Autodesk Inventor part; units mm, degrees
ref_plane "YZ Plane" through (0, 0, 0) normal (1, 0, 0) x (0, 1, 0)
ref_plane "XZ Plane" through (0, 0, 0) normal (0, 1, 0) x (-1, 0, 0)
ref_plane "XY Plane" through (0, 0, 0) normal (0, 0, 1) x (1, 0, 0)
sketch "card" plane through (0, 0, 0) normal (0, 0, 1) x (1, 0, 0)
  line L0 (-59.3579, 68.5808) -> (-59.3579, 10.0008)
  line L1 (-59.3579, 10.0008) -> (14.2921, 10.0008)
  line L2 (14.2921, 10.0008) -> (14.2921, 68.5808)
  line L3 (14.2921, 68.5808) -> (-59.3579, 68.5808)
  circle A0 centre (11.6671, 65.9558) radius 1.575
  circle A1 centre (11.6671, 12.6258) radius 1.575
  circle A2 centre (-56.7329, 65.9558) radius 1.575
  circle A3 centre (-56.7329, 12.6258) radius 1.575
  point P0 (0, 0)
  dimension "d1" = 58.58
  dimension "d2" = 73.65
  dimension "d4" = 2.625
  dimension "d5" = 3.15
extrude "main_board" add sketch "card" along normal blind 1.6
sketch "back_components" plane through (0, 0, 0) normal (0, 0, -1) x (-1, 0, 0)
  line L0 (-3.0921, 63.3708) -> (22.7279, 63.3708)
  line L1 (22.7279, 63.3708) -> (22.7279, 58.3708)
  line L2 (22.7279, 58.3708) -> (-3.0921, 58.3708)
  line L3 (-3.0921, 58.3708) -> (-3.0921, 63.3708)
  line L4 (-2.9921, 20.1008) -> (22.8179, 20.1008)
  line L5 (22.8179, 20.1008) -> (22.8179, 15.1008)
  line L6 (22.8179, 15.1008) -> (-2.9921, 15.1008)
  line L7 (-2.9921, 15.1008) -> (-2.9921, 20.1008)
  line L8 (-14.2921, 68.5808) -> (59.3579, 68.5808)
  line L9 (-14.2921, 10.0008) -> (-14.2921, 68.5808)
  line L10 (59.3579, 10.0008) -> (-14.2921, 10.0008)
  point P0 (0, 0)
  dimension "d23" = 5.21
  dimension "d24" = 11.2
  dimension "d25" = 5.1
  dimension "d26" = 11.3
  dimension "d27" = 5
  dimension "d28" = 5
  dimension "d29" = 25.82
  dimension "d30" = 25.81
extrude "pins_female" add sketch "back_components" along normal blind 8.37
extrude "pins_male1" add sketch "back_components" against normal blind 9.24 contours L0 L1 L2 L3
extrude "pins_male2" add sketch "back_components" against normal blind 9.24
sketch "front_components" plane through (0, 0, 1.6) normal (0, 0, 1) x (1, 0, 0)
  line L0 (-55.4979, 24.5008) -> (-61.1579, 24.5008)
  line L1 (-61.1579, 24.5008) -> (-61.1579, 16.5008)
  line L2 (-61.1579, 16.5008) -> (-55.4979, 16.5008)
  line L3 (-55.4979, 16.5008) -> (-55.4979, 24.5008)
  line L4 (-59.3579, 10.0008) -> (14.2921, 10.0008)
  line L5 (-59.3579, 68.5808) -> (-59.3579, 10.0008)
  line L6 (-35.1979, 60.9808) -> (-30.0979, 60.9808)
  line L7 (-30.0979, 60.9808) -> (-30.0979, 38.4308)
  line L8 (-30.0979, 38.4308) -> (-35.1979, 38.4308)
  line L9 (-35.1979, 38.4308) -> (-35.1979, 60.9808)
  line L10 (-32.0779, 22.0008) -> (-26.0779, 22.0008)
  line L11 (-26.0779, 22.0008) -> (-26.0779, 16.0008)
  line L12 (-26.0779, 16.0008) -> (-32.0779, 16.0008)
  line L13 (-32.0779, 16.0008) -> (-32.0779, 22.0008)
  line L14 (-22, 22) -> (-2, 22)
  line L15 (-2, 22) -> (-2, 16)
  line L16 (-2, 16) -> (-22, 16)
  line L17 (-22, 16) -> (-22, 22)
  line L18 (5.8421, 17.9408) -> (13.1421, 17.9408)
  line L19 (13.1421, 17.9408) -> (13.1421, 15.3408)
  line L20 (13.1421, 15.3408) -> (5.8421, 15.3408)
  line L21 (5.8421, 15.3408) -> (5.8421, 17.9408)
  line L22 (6.0921, 29.8608) -> (12.0921, 29.8608)
  line L23 (12.0921, 29.8608) -> (12.0921, 23.8608)
  line L24 (12.0921, 23.8608) -> (6.0921, 23.8608)
  line L25 (6.0921, 23.8608) -> (6.0921, 29.8608)
  line L26 (7.8321, 40.7108) -> (12.8321, 40.7108)
  line L27 (12.8321, 40.7108) -> (12.8321, 38.2308)
  line L28 (12.8321, 38.2308) -> (7.8321, 38.2308)
  line L29 (7.8321, 38.2308) -> (7.8321, 40.7108)
  line L30 (6.0921, 55.0808) -> (12.0921, 55.0808)
  line L31 (12.0921, 55.0808) -> (12.0921, 49.0808)
  line L32 (12.0921, 49.0808) -> (6.0921, 49.0808)
  line L33 (6.0921, 49.0808) -> (6.0921, 55.0808)
  line L34 (5.6421, 63.4208) -> (13.1421, 63.4208)
  line L35 (13.1421, 63.4208) -> (13.1421, 60.9408)
  line L36 (13.1421, 60.9408) -> (5.6421, 60.9408)
  line L37 (5.6421, 60.9408) -> (5.6421, 63.4208)
  line L38 (-27, 66) -> (-6, 66)
  line L39 (-6, 66) -> (-6, 62)
  line L40 (-6, 62) -> (-27, 62)
  line L41 (-27, 62) -> (-27, 66)
  line L42 (-32.0779, 26.1508) -> (-26.0779, 26.1508)
  line L43 (-26.0779, 26.1508) -> (-26.0779, 32.1508)
  line L44 (-26.0779, 32.1508) -> (-32.0779, 32.1508)
  line L45 (-32.0779, 32.1508) -> (-32.0779, 26.1508)
  line L46 (14.2921, 68.5808) -> (-59.3579, 68.5808)
  line L47 (14.2921, 10.0008) -> (14.2921, 68.5808)
  point P0 (0, 0)
  dimension "d19" = 6.5
  dimension "d20" = 8
  dimension "d21" = 1.8
  dimension "d22" = 5.66
  dimension "d31" = 27.28
  dimension "d32" = 6
  dimension "d33" = 6
  dimension "d34" = 6
  dimension "d35" = 4.15
  dimension "d36" = 6
  dimension "d37" = 6
  dimension "d38" = 5.16
  dimension "d39" = 2.48
  dimension "d40" = 5.86
  dimension "d41" = 6
  dimension "d42" = 6
  dimension "d43" = 8.37
  dimension "d44" = 2.48
  dimension "d45" = 7.5
  dimension "d46" = 6
  dimension "d47" = 6
  dimension "d48" = 8.37
  dimension "d49" = 5.92
  dimension "d50" = 2.6
  dimension "d51" = 1.15
  dimension "d58" = 7.6
  dimension "d59" = 22.55
  dimension "d60" = 5.1
  dimension "d61" = 24.16
  dimension "d62" = 2.2
  dimension "d63" = 1.46
  dimension "d64" = 5
  dimension "d65" = 7.3
  dimension "d66" = 1.15
extrude "vcc_gnd" add sketch "front_components" along normal blind 8.53 contours L18 L19 L20 L21 | L34 L35 L36 L37
extrude "buttons" add sketch "front_components" along normal blind 5 contours L10 L11 L12 L13 | L22 L23 L24 L25 | L30 L31 L32 L33 | L45 L44 L43 L42
extrude "sikring" add sketch "front_components" along normal blind 8.5 contours L6 L7 L8 L9 | L26 L27 L28 L29
extrude "micro_USB" add sketch "front_components" along normal blind 2.8 contours L3 L2 L5 L0 | L5 L2 L1 L0
properties part number "lunchpad"
Geometry check sheet. Reference: the model listing, model coordinates, mm. A direction names the side the tool comes from. Round coordinates to 2 decimals unless told otherwise and drop trailing zeros. Order: outer loops, then holes, each group sorted by start corner. A loop starts at its lowest first (then second) coordinate and runs counter-clockwise, first axis right, second up. Notation, with made-up numbers: (-34.5, 43) -> (0.5, 43) arc R17 cw to (0.5, 54) -> close; hole circle Ø8 at (28, 67.5). An arc over 180 degrees is marked (long way). Return JSON: item names as keys, results as strings. Group by question number.
Q1. Section check C-C, the plane x = -11. Record the boundary of the cut face in (y, z), plus the area to 3 significant figures.
Q2. Material ranges on probe 1 along Y at (x, z) = (7.5, 3.25); probe 2 along X at (y, z) = (52.5, 2.5); probe 3 along X at (y, z) = (61.5, 5.75), recorded low to high. Write a range as from..to.
Q3. Section check B-B, the plane y = 29. Record the boundary of the cut face in (x, z), plus the area to 3 significant figures.
Q4. Section check A-A, the plane z = -6. Record the boundary of the cut face in (x, y), plus the area to 3 significant figures.
Q5. Release check for a two-part mould opening along Y. For faces 5 (the flat face through (-10, 63.371, -4)), 6 (the flat face through (-61.158, 21, 3)), 7 (the flat face through (9, 49.081, 4)) record: released by +Y, released by -Y, zero draft, split by the parting line, or undercut.
Q6. Gauge pin test, flat ends, axial feed: pin 1 (3 mm diameter, centred on x = -56.73, y = 12.63, fed in from +Z); pin 2 (1.5 mm diameter, centred on y = 41.5, z = 2.5, fed in from -X); pin 3 (2.5 mm diameter, centred on x = -15, z = 7, fed in from +Y); pin 4 (3 mm diameter, centred on x = 5.5, y = 50, fed in from +Z). Record the tip position at first contact, or that the pin passes through.
Q7. Tool access check on faces 1 (the flat face through (5.842, 17, 6)), 2 (the flat face through (10, 40.711, 6)), 3 (the flat face through (-58, 21, 4.4)), 4 (the flat face through (2.992, 18, -4)). Record the directions out of +Z, -Z, +X, -X, +Y, -Y that give a thin tool (end or side, any length) a straight path to the whole face; none if there is none.
Q8. Section check D-D, the plane z = 3.5. Count the separate pieces of the cut face and the enclosed holes in it, plus the area to 3 significant figures.
Numbers:
{
 "1": {"outline": "(10, 0) -> (15.1, 0) -> (15.1, -8.37) -> (20.1, -8.37) -> (20.1, 0) -> (58.37, 0) -> (58.37, -8.37) -> (63.37, -8.37) -> (63.37, 0) -> (68.58, 0) -> (68.58, 1.6) -> (63.37, 1.6) -> (63.37, 9.24) -> (58.37, 9.24) -> (58.37, 1.6) -> (20.1, 1.6) -> (20.1, 9.24) -> (15.1, 9.24) -> (15.1, 1.6) -> (10, 1.6) -> close", "area": "254 mm^2"},
 "2": {"probe 1": "15.34..17.94, 23.86..29.86, 49.08..55.08, 60.94..63.42", "probe 2": "-35.2..-30.1, 6.09..12.09", "probe 3": "-22.73..3.09, 5.64..13.14"},
 "3": {"outline": "(-59.36, 0) -> (14.29, 0) -> (14.29, 1.6) -> (12.09, 1.6) -> (12.09, 6.6) -> (6.09, 6.6) -> (6.09, 1.6) -> (-26.08, 1.6) -> (-26.08, 6.6) -> (-32.08, 6.6) -> (-32.08, 1.6) -> (-59.36, 1.6) -> close", "area": "178 mm^2"},
 "4": {"outline": "(-22.82, 15.1) -> (2.99, 15.1) -> (2.99, 20.1) -> (-22.82, 20.1) -> close; (-22.73, 58.37) -> (3.09, 58.37) -> (3.09, 63.37) -> (-22.73, 63.37) -> close", "area": "258 mm^2"},
 "5": {"face 5": "released by +Y", "face 6": "zero draft", "face 7": "undercut"},
 "6": {"pin 1": "through", "pin 2": "x = -35.2", "pin 3": "y = 63.37", "pin 4": "z = 6.6"},
 "7": {"face 1": "+Z, -Y", "face 2": "+Z, +X", "face 3": "+Z, -X, +Y, -Y", "face 4": "-Z, +X, -Y"},
 "8": {"separate pieces": "11", "enclosed holes": "0", "area": "612 mm^2"}
}
